from build123d import *
from OCP.BRepFilletAPI import BRepFilletAPI_MakeChamfer

# Parameters (mm, degrees)
SKETCH2_W                                    = 60
SKETCH2_H                                    = 44.3
SKETCH2_R                                    = 2.25
SKETCH2_R_2                                  = 7.75
BOSS_EXTRUDE1_DEPTH                          = 5
CBORE_FOR_M4_HEX_SOCKET_HEAD_CAP_SCR_2_COUNT = 2
CBORE_FOR_M4_HEX_SOCKET_HEAD_CAP_SCR_2_PITCH = 40
CBORE_FOR_M4_HEX_SOCKET_HEAD_CAP_SCR_3_COUNT = 2
CBORE_FOR_M4_HEX_SOCKET_HEAD_CAP_SCR_3_PITCH = 48.826222463
CBORE_FOR_M4_HEX_SOCKET_HEAD_CAP_SCR_4_COUNT = 2
CBORE_FOR_M4_HEX_SOCKET_HEAD_CAP_SCR_4_PITCH = 28
SKETCH7_R                                    = 11.1
CUT_EXTRUDE1_DEPTH                           = 2.7
CHAMFER2_SIZE                                = 22
CHAMFER2_SIZE2                               = 8.007345154
CHAMFER3_SIZE                                = 2
CHAMFER1_SIZE                                = 5


with BuildPart() as part:
    # Sketch2 → Boss-Extrude1 (new body)
    with BuildSketch(Plane.XY):
        Rectangle(SKETCH2_W, SKETCH2_H)
        with Locations((-20, 14)):
            Circle(SKETCH2_R, mode=Mode.SUBTRACT)
        with Locations((-20, -14)):
            Circle(SKETCH2_R, mode=Mode.SUBTRACT)
        with Locations((20, 14)):
            Circle(SKETCH2_R, mode=Mode.SUBTRACT)
        with Locations((20, -14)):
            Circle(SKETCH2_R, mode=Mode.SUBTRACT)
        with Locations((-8.2, 0)):
            Circle(SKETCH2_R_2, mode=Mode.SUBTRACT)
    extrude(amount=BOSS_EXTRUDE1_DEPTH)

    # Sketch4 → CBORE for M4 Hex Socket Head Cap Screw1 (revolve, cut)
    with BuildSketch(Plane(origin=(-20, 14, 5), x_dir=(0, -1, 0), z_dir=(1, 0, 0))):
        Polygon((0, 0), (0, 5), (2.25, 5), (2.25, 1), (4, 1), (4, 0.025), (4.025, 0), align=None)
    cbore_for_m4_hex_socket_head_cap_screw1 = revolve(axis=Axis((-20, 14, 11.35), (0, 0, -1)), mode=Mode.SUBTRACT)

    # CBORE for M4 Hex Socket Head Cap Scr 2: CBORE for M4 Hex Socket Head Cap Screw1 ×2
    with Locations(*[(i * CBORE_FOR_M4_HEX_SOCKET_HEAD_CAP_SCR_2_PITCH, 0, 0) for i in range(1, CBORE_FOR_M4_HEX_SOCKET_HEAD_CAP_SCR_2_COUNT)]):
        add(cbore_for_m4_hex_socket_head_cap_screw1, mode=Mode.SUBTRACT)

    # CBORE for M4 Hex Socket Head Cap Scr 3: CBORE for M4 Hex Socket Head Cap Screw1 ×2
    with Locations(*[Vector(0.8192319205190405, -0.5734623443633283, 0) * (i * CBORE_FOR_M4_HEX_SOCKET_HEAD_CAP_SCR_3_PITCH) for i in range(1, CBORE_FOR_M4_HEX_SOCKET_HEAD_CAP_SCR_3_COUNT)]):
        add(cbore_for_m4_hex_socket_head_cap_screw1, mode=Mode.SUBTRACT)

    # CBORE for M4 Hex Socket Head Cap Scr 4: CBORE for M4 Hex Socket Head Cap Screw1 ×2
    with Locations(*[(0, -i * CBORE_FOR_M4_HEX_SOCKET_HEAD_CAP_SCR_4_PITCH, 0) for i in range(1, CBORE_FOR_M4_HEX_SOCKET_HEAD_CAP_SCR_4_COUNT)]):
        add(cbore_for_m4_hex_socket_head_cap_screw1, mode=Mode.SUBTRACT)

    # Sketch7 → Cut-Extrude1 (cut)
    with BuildSketch(Plane(origin=(0, 0, 0), x_dir=(-1, 0, 0), z_dir=(0, 0, -1))):
        with Locations((8.2, 0)):
            Circle(SKETCH7_R)
    extrude(amount=-CUT_EXTRUDE1_DEPTH, mode=Mode.SUBTRACT)

    # Chamfer2: one chamfer whose edges measure the first distance from different faces: ONE call of the kernel's chamfer builder (chamfer() names one face for all edges)
    chamfer2_edges_1 = [part.edges().sort_by_distance(p)[0] for p in [
        (-30, 22.15, 2.5),
    ]]
    chamfer2_side_1 = [part.faces().sort_by_distance(p)[0] for p in [
        (-30, 0, 2.5),
    ]]
    chamfer2_edges_2 = [part.edges().sort_by_distance(p)[0] for p in [
        (30, 22.15, 2.5),
    ]]
    chamfer2_side_2 = [part.faces().sort_by_distance(p)[0] for p in [
        (30, 0, 2.5),
    ]]
    chamfer2 = BRepFilletAPI_MakeChamfer(part.part.solid().wrapped)
    for e in chamfer2_edges_1:
        chamfer2.Add(CHAMFER2_SIZE, CHAMFER2_SIZE2, e.wrapped, chamfer2_side_1[0].wrapped)  # the first distance lies on this face
    for e in chamfer2_edges_2:
        chamfer2.Add(CHAMFER2_SIZE, CHAMFER2_SIZE2, e.wrapped, chamfer2_side_2[0].wrapped)  # the first distance lies on this face
    add(Compound.cast(chamfer2.Shape()), mode=Mode.REPLACE)

    # Chamfer3
    chamfer3_edges = [part.edges().sort_by_distance(p)[0] for p in [
        (0, -22.15, 5),
        (0, 22.15, 5),
    ]]
    chamfer(chamfer3_edges, length=CHAMFER3_SIZE)

    # Chamfer1
    chamfer1_edges = [part.edges().sort_by_distance(p)[0] for p in [
        (-30, -11, 0),
        (30, -11, 0),
    ]]
    chamfer(chamfer1_edges, length=CHAMFER1_SIZE - 0.0001)  # a hair under: the kernel refuses the full size


solid = part.part
Design review of the part built by this model. Coordinates are the model's own, in mm. A direction names the side the tool comes from. Coordinates: 2 decimals unless noted, no trailing zeros. Write each loop counter-clockwise with the first axis right and the second up, starting at its lowest first coordinate (ties: lowest second). Pieces come first, ordered by that corner, then holes. Notation, with made-up numbers: (-26, 42) - (16, 42) arc R21 ccw to (16, 63) - close; hole circle Ø4 at (44, -0.5). An arc over 180 degrees is marked (long way). Use one line per item in the form item = value.
Q1. Insertion check: pin 1 Ø2 at (y, z) = (12.5, 1.5) entering from +X; pin 2 Ø11 at (x, y) = (-5, 3) entering from -Z. Each pin has a flat end and moves straight along its axis. Give the tip position at first contact, or say it passes through.
Taken from the geometry:
pin_1 = 25.87
pin_2 = 2.7
Q2. The part is to be moulded in two halves that separate along X. For faces 1 (the flat face through (-25.05, 13.75, 3.02)), 2 (the flat face through (28, -8, 3)), 3 (the cylindrical face through (-22.7, 16.95, 4.49)), 4 (the cylindrical face through (19.512, 11.804, 1.972)), say which applies: +X half, -X half, draft (parallel to the pull), parting line (faces both ways), or undercut.
Taken from the geometry:
face_1 = -X half
face_2 = +X half
face_3 = undercut
face_4 = undercut
Q3. Consider section C-C (x = -2). Write out the cut boundary in (y, z).
Taken from the geometry:
outline = (-22.15, 0) - (-9.21, 0) - (-9.21, 2.7) - (-4.65, 2.7) - (-4.65, 5) - (-20.15, 5) - (-22.15, 3) - close; (4.65, 2.7) - (9.21, 2.7) - (9.21, 0) - (22.15, 0) - (22.15, 3) - (20.15, 5) - (4.65, 5) - close
Q4. Machinability: for faces 5 (the cylindrical face through (22.4, -10.8, 4.5)), 6 (the flat face through (-11, 8, 2.7)), 7 (the cylindrical face through (-20.488, 11.804, 1.972)), which of the approach directions +Z, -Z, +X, -X, +Y, -Y give a long, thin tool a straight path to every point of the face, cutting with its end or side? Answer none if there is none.
Taken from the geometry:
face_5 = +Z
face_6 = -Z
face_7 = +Z, -Z
Q5. For probe 1 along Y at (x, z) = (20, 1.55); probe 2 along X at (y, z) = (-13.5, 2.9); probe 3 along X at (y, z) = (-12, 1.7), list the stretches that pass through material, from the lowest coordinate up.
Taken from the geometry:
probe_1 = -22.15 to -16.25, -11.75 to 11.75, 16.25 to 22.15
probe_2 = -27.9 to -22.19, -17.81 to 17.81, 22.19 to 27.9
probe_3 = -26.7 to -21.03, -18.97 to 18.97, 21.03 to 26.7
Q6. Consider section B-B (y = -14). Count the separate pieces of the cut face and the enclosed holes in it, plus the area to 3 significant figures.
Taken from the geometry:
separate_pieces = 3
enclosed_holes = 0
area = 223 mm^2
Q7. Consider section A-A (x = 20). Write out the cut boundary in (y, z) (3 decimals), plus the area to 3 significant figures.
Taken from the geometry:
outline = (-22.15, 0) - (-16.25, 0) - (-16.25, 4) - (-18, 4) - (-18, 4.975) - (-18.025, 5) - (-20.15, 5) - (-22.15, 3) - close; (-11.75, 0) - (11.75, 0) - (11.75, 4) - (10, 4) - (10, 4.975) - (9.975, 5) - (-9.975, 5) - (-10, 4.975) - (-10, 4) - (-11.75, 4) - close; (16.25, 0) - (22.15, 0) - (22.15, 3) - (20.15, 5) - (18.025, 5) - (18, 4.975) - (18, 4) - (16.25, 4) - close
area = 165 mm^2
Q8. Consider section D-D (z = 1.9). Write out the cut boundary in (x, y).
Taken from the geometry:
outline = (-26.9, -22.15) - (26.9, -22.15) - (26.9, 8.67) - (21.99, 22.15) - (-21.99, 22.15) - (-26.9, 8.67) - close; hole circle Ø4.5 at (-20, -14); hole circle Ø4.5 at (-20, 14); hole circle Ø22.2 at (-8.2, 0); hole circle Ø4.5 at (20, -14); hole circle Ø4.5 at (20, 14)
